from build123d import *

# Parameters (mm, degrees)
F1_DEPTH = 15
F2_W     = 33
F2_H     = 58
F3_DEPTH = 15.001


with BuildPart() as f1:
    # F0 (on Top) → F1 (new body)
    with BuildSketch(Plane.XY):
        with BuildLine():
            Line((-100, -250), (100, -250))
            ThreePointArc((100, -250), (135.355339, -235.355339), (150, -200))
            Line((150, -200), (150, 100))
            ThreePointArc((150, 100), (0, 250), (-150, 100))
            Line((-150, 100), (-150, -200))
            ThreePointArc((-150, -200), (-135.355339, -235.355339), (-100, -250))
        make_face()
    extrude(amount=F1_DEPTH)

    # F2 (on face) → F3 (cut, through all)
    with BuildSketch(Plane.XY.offset(15)):
        with Locations((0, 44)):
            Rectangle(F2_W, F2_H)
    extrude(amount=-F3_DEPTH, mode=Mode.SUBTRACT)


solid = f1.part
For this review, take the finished solid that the model builds, in its own axes (mm). A direction names the side the tool comes from. Coordinates: 2 decimals unless noted, no trailing zeros. Order: outer loops, then holes, each group sorted by start corner. A loop starts at its lowest first (then second) coordinate and runs counter-clockwise, first axis right, second up. Notation, with made-up numbers: (77, 82) -> (100, 82) arc R11 cw to (100, 101) -> close; hole circle Ø10 at (-17, 88.25). An arc over 180 degrees is marked (long way). Return JSON: item names as keys, results as strings.
1. We need section D-D on x = -75. Write out the cut boundary in (y, z).
Answer block:
{"outline": "(-250, 0) -> (229.9, 0) -> (229.9, 15) -> (-250, 15) -> close"}
2. We need section C-C on y = 191. Write out the cut boundary in (x, z).
Answer block:
{"outline": "(-119.24, 0) -> (119.24, 0) -> (119.24, 15) -> (-119.24, 15) -> close"}
3. We need section B-B on z = 12.75. Write out the cut boundary in (x, y), and give its area (3 significant figures).
Answer block:
{"outline": "(-150, -200) arc R50 ccw to (-100, -250) -> (100, -250) arc R50 ccw to (150, -200) -> (150, 100) arc R150 ccw to (-150, 100) -> close; hole (-16.5, 15) -> (16.5, 15) -> (16.5, 73) -> (-16.5, 73) -> close", "area": "137,000 mm²"}
4. For pin 1 Ø5 at (x, z) = (106, 11.5) entering from -Y; pin 2 Ø3 at (y, z) = (195, 8.5) entering from -X; pin 3 Ø6 at (x, y) = (-36.5, 164) entering from -Z, all flat-tipped, find the tip position at first contact; note any pin that passes through.
Answer block:
{"pin 1": "y = -249.88", "pin 2": "x = -117.29", "pin 3": "z = 0"}
5. Machinability: for faces 4 (the flat face through (-150, -48, 7)), 5 (the flat face through (0, 73, 8)), which of the approach directions +Z, -Z, +X, -X, +Y, -Y give a long, thin tool a straight path to every point of the face, cutting with its end or side? Answer none if there is none.
Answer block:
{"face 4": "+Z, -Z, -X, +Y, -Y", "face 5": "+Z, -Z"}
6. The part is to be moulded in two halves that separate along Y. For faces 1 (the flat face through (-2, 4, 0)), 2 (the cylindrical face through (3.298, 249.964, 7.395)), 3 (the flat face through (-16.5, 44, 8)), say which applies: +Y half, -Y half, draft (parallel to the pull), parting line (faces both ways), or undercut.
Answer block:
{"face 1": "draft", "face 2": "+Y half", "face 3": "undercut"}
7. We need section A-A on x = 0. Write out the cut boundary in (y, z).
Answer block:
{"outline": "(-250, 0) -> (15, 0) -> (15, 15) -> (-250, 15) -> close; (73, 0) -> (250, 0) -> (250, 15) -> (73, 15) -> close"}
8. For line 1 (X direction, y = -200.5, z = 3.5); line 2 (Y direction, x = -65, z = 9.75); line 3 (Y direction, x = -51.5, z = 13.5), list the stretches that pass through material, from the lowest coordinate up. Write a range as from..to.
Answer block:
{"line 1": "-150..150", "line 2": "-250..235.19", "line 3": "-250..240.88"}
